The model under review builds one solid part; all positions refer to its coordinate system, in mm. Coordinates: 2 decimals unless noted, no trailing zeros. Write each loop counter-clockwise with the first axis right and the second up, starting at its lowest first coordinate (ties: lowest second). Pieces come first, ordered by that corner, then holes. Notation, with made-up numbers: (-23, -20) - (13, -20) arc R21 cw to (13, 2) - close; hole circle Ø2 at (29.25, 59.5). An arc over 180 degrees is marked (long way). Put each result on its own line as item: value. Start each with the question number.
Item 1: Consider section A-A on z = -11. Give the boundary of the cut face in (x, y), then the cut area to 3 significant figures.
Item 2: Consider section C-C on y = 115.5. Give the boundary of the cut face in (x, z).
Item 3: For pin 1 (5 mm diameter, centred on x = -95.5, y = 53, fed in from -Z); pin 2 (2 mm diameter, centred on y = 56.5, z = 10.5, fed in from +X); pin 3 (8 mm diameter, centred on y = 116, z = -27.5, fed in from +X), all flat-tipped, find the tip position at first contact; note any pin that passes through.
Item 4: To check wall thickness, follow L1, parallel to X at y = 83.5, z = -15; L2, parallel to X at y = 37, z = 10; L3, parallel to X at y = 11.5, z = -24. State the ranges of each line that lie inside material, in increasing order. Write a range as [from, to].
Item 5: Consider section B-B on z = -30. Give the boundary of the cut face in (x, y), then the cut area to 3 significant figures.
Item 6: Consider section D-D on x = 39. Give the boundary of the cut face in (y, z).
```python
from build123d import *

# Parameters (mm, degrees)
EXTRUDE_1_DEPTH = 135


with BuildPart() as part:
    # Эскиз4 → Бобышка-Вытянуть1 (new body)
    with BuildSketch(Plane(origin=(0, 0, 0), x_dir=(1, 0, 0), z_dir=(0, 1, 0))):
        with BuildLine():
            Line((110.708418771, 22.141683754), (115.702479941, 23.140495988))
            ThreePointArc((115.702479941, 23.140495988), (67.475569561, -36.55139996), (0, 0))
            ThreePointArc((0, 0), (-67.475569561, 36.55139996), (-115.702479941, -23.140495988))
            Line((-115.702479941, -23.140495988), (-120.682183817, -24.136436763))
            ThreePointArc((-120.682183817, -24.136436763), (-68.909214493, 41.362013423), (4.642383454, 1.856953382))
            ThreePointArc((4.642383454, 1.856953382), (66.039906911, -31.737519495), (110.708418771, 22.141683754))
        make_face()
    extrude(amount=EXTRUDE_1_DEPTH)


solid = part.part
```
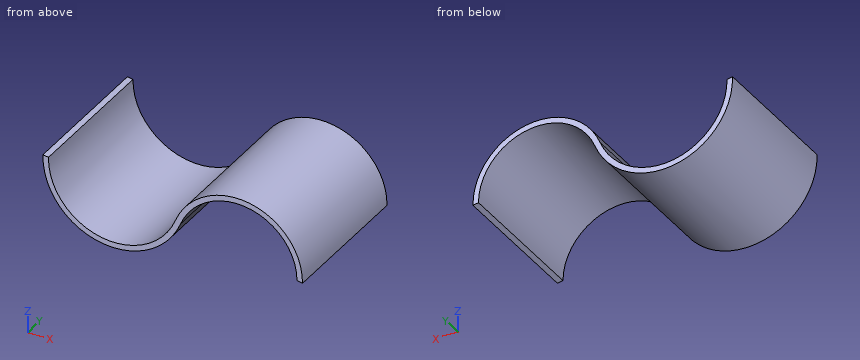
Report:
1. outline: (-111.54, 0) - (-105.63, 0) - (-105.63, 135) - (-111.54, 135) - close; (-5.79, 0) - (0.12, 0) - (0.12, 135) - (-5.79, 135) - close; (109.54, 0) - (114.64, 0) - (114.64, 135) - (109.54, 135) - close
1. area: 2,280 mm²
2. outline: (-120.68, 24.14) arc R65 ccw to (4.64, -1.86) arc R55 cw to (110.71, -22.14) - (115.7, -23.14) arc R60 ccw to (0, 0) arc R60 cw to (-115.7, 23.14) - close
3. pin 1: z = -30.96
3. pin 2: x = 106.6
3. pin 3: x = -9.57
4. L1: [-108.95, -102.72], [-8.7, -2.46], [110.22, 115.26]
4. L2: [-119.54, -114.44], [5.13, 11.18], [100.24, 106.28]
4. L3: [-101.35, -93.89], [-17.53, -10.07]
5. outline: (-94.33, 0) - (-85.14, 0) - (-85.14, 135) - (-94.33, 135) - close; (-26.27, 0) - (-17.09, 0) - (-17.09, 135) - (-26.27, 135) - close
5. area: 2,480 mm²
6. outline: (0, 30.12) - (135, 30.12) - (135, 35.34) - (0, 35.34) - close
